Design review of the part built by this model. Coordinates are the model's own, in mm. Give positions to 0.01 mm unless a question says otherwise; leave off trailing zeros. Order: outer loops, then holes, each group sorted by start corner. A loop starts at its lowest first (then second) coordinate and runs counter-clockwise, first axis right, second up.
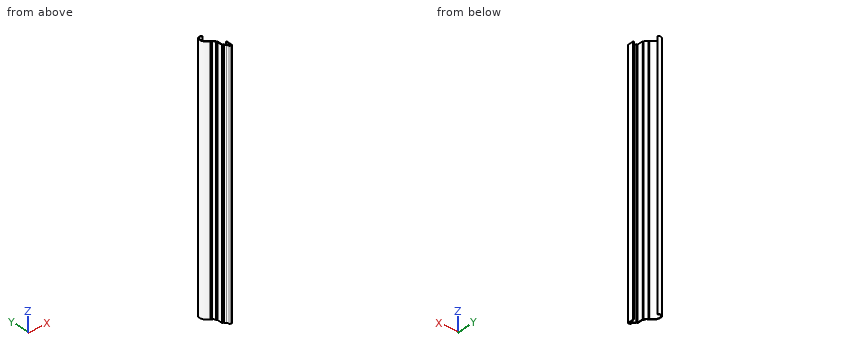
```python
from build123d import *

# Parameters (mm, degrees)
EXTRUDE_THIN1_DEPTH = 492.125
FILLET1_R           = 1.27


with BuildPart() as part:
    # Sketch1 → Extrude-Thin1 (new body)
    with BuildSketch(Plane.XY):
        with BuildLine():
            Line((0, 0), (0, -12.7))
            Line((0, -12.7), (-5.159375, -12.7))
            Line((-5.159375, -12.7), (-5.159375, -10.842826643))
            ThreePointArc((-5.159375, -10.842826643), (-5.691086679, -8.858451643), (-7.14375, -7.405788321))
            ThreePointArc((-7.14375, -7.405788321), (-8.596413321, -5.953125), (-9.128125, -3.96875))
            Line((-9.128125, -3.96875), (-11.90625, -3.96875))
            Line((-11.90625, -3.96875), (-11.90625, 7.9375))
            Line((-11.90625, 7.9375), (-13.49375, 7.9375))
            Line((-13.49375, 7.9375), (-13.49375, 10.240343132))
            ThreePointArc((-13.49375, 10.240343132), (-15.016214309, 13.124180094), (-18.25625, 13.49375))
            Line((-18.25625, 13.49375), (-18.25625, 15.875))
            ThreePointArc((-18.25625, 15.875), (-26.477500212, 21.947406572), (-28.305018694, 32.003412381))
            ThreePointArc((-28.305018694, 32.003412381), (-23.995750741, 36.384342306), (-18.25625, 34.18878576))
            Line((-18.25625, 34.18878576), (-19.28547828, 33.444750043))
            ThreePointArc((-19.28547828, 33.444750043), (-23.725863862, 35.143350335), (-27.059744656, 31.754027996))
            ThreePointArc((-27.059744656, 31.754027996), (-25.135637157, 22.212936626), (-16.98625, 16.891085148))
            Line((-16.98625, 16.891085148), (-16.98625, 15.002843132))
            ThreePointArc((-16.98625, 15.002843132), (-13.618653955, 13.607939177), (-12.22375, 10.240343132))
            Line((-12.22375, 10.240343132), (-12.22375, 9.2075))
            Line((-12.22375, 9.2075), (-10.63625, 9.2075))
            Line((-10.63625, 9.2075), (-10.63625, -2.69875))
            Line((-10.63625, -2.69875), (-7.540625, -2.69875))
            ThreePointArc((-7.540625, -2.69875), (-7.754050035, -4.710985155), (-6.50875, -6.305936058))
            ThreePointArc((-6.50875, -6.305936058), (-4.591234416, -8.223451643), (-3.889375, -10.842826643))
            Line((-3.889375, -10.842826643), (-3.889375, -11.43))
            Line((-3.889375, -11.43), (-1.27, -11.43))
            Line((-1.27, -11.43), (-1.27, 0))
            Line((-1.27, 0), (0, 0))
        make_face()
    extrude(amount=-EXTRUDE_THIN1_DEPTH)

    # Fillet1
    fillet1_edges = [part.edges().sort_by_distance(p)[0] for p in [
        (-16.98625, 16.891085148, -246.0625),
        (-10.63625, 9.2075, -246.0625),
        (-7.540625, -2.69875, -246.0625),
        (0, -12.7, -246.0625),
        (-5.159375, -12.7, -246.0625),
        (-11.90625, -3.96875, -246.0625),
        (-13.49375, 7.9375, -246.0625),
        (-18.25625, 13.49375, -246.0625),
    ]]
    fillet(fillet1_edges, radius=FILLET1_R)


solid = part.part
```
1. For line 1 along X through (y, z) = (30.5, -104.5); line 2 along Y through (x, z) = (-21.25, -378.5); line 3 along X through (y, z) = (7, -215), list the stretches that pass through material, from the lowest coordinate up.
Recorded:
line 1: x = -28.52 to -27.25
line 2: y = 17.05 to 18.52, 34.96 to 36.29
line 3: x = -11.91 to -10.64
2. Take a section at A-A (y = 23). State the section outline as (x, z) points (3 decimals).
Recorded:
outline: (-27.071, -492.125) - (-25.628, -492.125) - (-25.628, 0) - (-27.071, 0) - close
3. For pin 1 (3 mm diameter, centred on x = -24, y = 29.5, fed in from +Z); pin 2 (0.8 mm diameter, centred on x = -10, z = -334, fed in from -Y); pin 3 (5 mm diameter, centred on x = -13.5, z = -102, fed in from +Y); pin 4 (0.6 mm diameter, centred on y = -11, z = -291, fed in from -X), all flat-tipped, find the tip position at first contact; note any pin that passes through.
Recorded:
pin 1: passes through
pin 2: stops at y = -3.97
pin 3: stops at y = 14.9
pin 4: stops at x = -5.16
